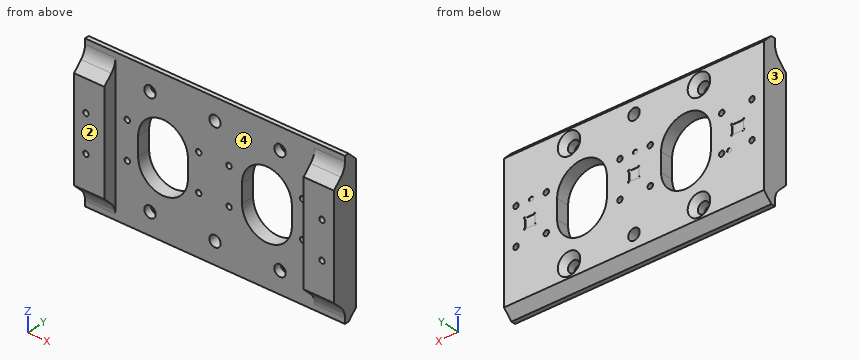
```python
from build123d import *

# Parameters (mm, degrees)
SKETCH_5_W                  = 120
SKETCH_5_H                  = 70
EXTRUDE_2_DEPTH             = 6
SKETCH1_R                   = 1
CUT_EXTRUDE1_DEPTH          = 0.2
SKETCH2_R                   = 1
CUT_EXTRUDE2_DEPTH          = 0.2
HOLE_WIZARD_M51_D           = 5.3
HOLE_WIZARD_M51_CSINK_D     = 10.4
HOLE_WIZARD_M51_CSINK_ANGLE = 90
SKETCH5_R                   = 2.6
CUT_EXTRUDE4_DEPTH          = 10
CUT_EXTRUDE4_TAPER          = -0.573055556
CUT_EXTRUDE_1_DEPTH         = 7.0000001
EXTRUDE_3_DEPTH             = 120
SKETCH_8_W                  = 92
SKETCH_8_H                  = 35.619722669
CUT_EXTRUDE_2_DEPTH         = 71
CHAMFER_1_SIZE              = 4
M3X0_51_D                   = 2.5


with BuildPart() as part:
    # Эскиз5 → Бобышка-Вытянуть2 (new body)
    with BuildSketch(Plane(origin=(0, 0, 0), x_dir=(1, 0, 0), z_dir=(0, 1, 0))):
        with Locations((60, 0)):
            Rectangle(SKETCH_5_W, SKETCH_5_H)
    extrude(amount=-EXTRUDE_2_DEPTH)

    # Sketch1 → Cut-Extrude1 (cut)
    with BuildSketch(Plane(origin=(0, 0, 0), x_dir=(1, 0, 0), z_dir=(0, 1, 0))):
        with Locations((16, 8)):
            Circle(SKETCH1_R)
        with BuildLine():
            Line((9.86, -2.16), (14.14, -2.16))
            ThreePointArc((14.14, -2.16), (14.993553391, -2.513553391), (14.64, -1.66))
            Line((14.64, -1.66), (14.64, 1.66))
            ThreePointArc((14.64, 1.66), (14.993553391, 2.513553391), (14.14, 2.16))
            Line((14.14, 2.16), (9.86, 2.16))
            ThreePointArc((9.86, 2.16), (9.006446609, 2.513553391), (9.36, 1.66))
            Line((9.36, 1.66), (9.36, -1.66))
            ThreePointArc((9.36, -1.66), (9.006446609, -2.513553391), (9.86, -2.16))
        make_face()
    extrude(amount=-CUT_EXTRUDE1_DEPTH, mode=Mode.SUBTRACT)

    # Sketch2 → Cut-Extrude2 (cut)
    with BuildSketch(Plane(origin=(0, 0, 0), x_dir=(1, 0, 0), z_dir=(0, 1, 0))):
        with Locations((59.481, -9.027)):
            Circle(SKETCH2_R)
        with Locations((107.481, -9.027)):
            Circle(SKETCH2_R)
        with BuildLine():
            Line((57.74, 1.76), (57.74, -1.76))
            ThreePointArc((57.74, -1.76), (57.386446609, -2.613553391), (58.24, -2.26))
            Line((58.24, -2.26), (61.76, -2.26))
            ThreePointArc((61.76, -2.26), (62.613553391, -2.613553391), (62.26, -1.76))
            Line((62.26, -1.76), (62.26, 1.76))
            ThreePointArc((62.26, 1.76), (62.613553391, 2.613553391), (61.76, 2.26))
            Line((61.76, 2.26), (58.24, 2.26))
            ThreePointArc((58.24, 2.26), (57.386446609, 2.613553391), (57.74, 1.76))
        make_face()
        with BuildLine():
            Line((105.74, 1.76), (105.74, -1.76))
            ThreePointArc((105.74, -1.76), (105.386446609, -2.613553391), (106.24, -2.26))
            Line((106.24, -2.26), (109.76, -2.26))
            ThreePointArc((109.76, -2.26), (110.613553391, -2.613553391), (110.26, -1.76))
            Line((110.26, -1.76), (110.26, 1.76))
            ThreePointArc((110.26, 1.76), (110.613553391, 2.613553391), (109.76, 2.26))
            Line((109.76, 2.26), (106.24, 2.26))
            ThreePointArc((106.24, 2.26), (105.386446609, 2.613553391), (105.74, 1.76))
        make_face()
    extrude(amount=-CUT_EXTRUDE2_DEPTH, mode=Mode.SUBTRACT)

    # Зенковка для  винта с плоской головкой M51 (through all)
    with Locations(Plane(origin=(0, 0, 0), x_dir=(1, 0, 0), z_dir=(0, 1, 0))):
        with Locations((30, 25), (90, 25), (90, -25), (30, -25)):
            CounterSinkHole(HOLE_WIZARD_M51_D / 2, HOLE_WIZARD_M51_CSINK_D / 2, counter_sink_angle=HOLE_WIZARD_M51_CSINK_ANGLE)

    # Sketch5 → Cut-Extrude4 (cut)
    with BuildSketch(Plane.XZ.offset(6)):
        with Locations((60, 25)):
            Circle(SKETCH5_R)
        with Locations((60, -25)):
            Circle(SKETCH5_R)
    extrude(amount=-CUT_EXTRUDE4_DEPTH, taper=CUT_EXTRUDE4_TAPER, mode=Mode.SUBTRACT)

    # Эскиз6 → Вырез-Вытянуть1 (cut, through all)
    with BuildSketch(Plane(origin=(0, 0, 0), x_dir=(1, 0, 0), z_dir=(0, 1, 0))):
        with BuildLine():
            Line((95.5, 4.35), (95.5, -4.35))
            ThreePointArc((95.5, -4.35), (84, -15.85), (72.5, -4.35))
            Line((72.5, -4.35), (72.5, 4.35))
            ThreePointArc((72.5, 4.35), (84, 15.85), (95.5, 4.35))
        make_face()
        with BuildLine():
            Line((47.5, 4.35), (47.5, -4.35))
            ThreePointArc((47.5, -4.35), (36, -15.85), (24.5, -4.35))
            Line((24.5, -4.35), (24.5, 4.35))
            ThreePointArc((24.5, 4.35), (36, 15.85), (47.5, 4.35))
        make_face()
    extrude(amount=-CUT_EXTRUDE_1_DEPTH, mode=Mode.SUBTRACT)

    # Эскиз7 → Бобышка-Вытянуть3 (add, through all)
    with BuildSketch(Plane.ZY):
        with BuildLine():
            Line((-32.5, -6), (32.5, -6))
            ThreePointArc((32.5, -6), (29.629874257, -6.570903506), (27.196699141, -8.196699141))
            Line((27.196699141, -8.196699141), (23.393398282, -12))
            Line((23.393398282, -12), (-23.393398282, -12))
            Line((-23.393398282, -12), (-27.196699141, -8.196699141))
            ThreePointArc((-27.196699141, -8.196699141), (-29.629874257, -6.570903506), (-32.5, -6))
        make_face()
    extrude(amount=-EXTRUDE_3_DEPTH)

    # Эскиз8 → Вырез-Вытянуть2 (cut, through all)
    with BuildSketch(Plane(origin=(0, 0, -35), x_dir=(-1, 0, 0), z_dir=(0, 0, -1))):
        with Locations((-60, -23.809861335)):
            Rectangle(SKETCH_8_W, SKETCH_8_H)
    extrude(amount=-CUT_EXTRUDE_2_DEPTH, mode=Mode.SUBTRACT)

    # Фаска1
    chamfer_1_edges = [part.edges().sort_by_distance(p)[0] for p in [
        (60, 0, 35),
        (60, 0, -35),
    ]]
    chamfer(chamfer_1_edges, length=CHAMFER_1_SIZE)

    # Отверстие обработанное метчиком M3x0.51 (through all)
    with Locations(Plane(origin=(0, 0, 0), x_dir=(1, 0, 0), z_dir=(0, 1, 0))):
        with Locations((114.481, -9.027), (100.481, -9.027), (100.481, 7.973), (114.481, 7.973), (66.481, 7.973), (52.481, 7.973), (52.481, -9.027), (66.481, -9.027), (19.5, -9), (5.5, -9), (5.5, 8), (19.5, 8)):
            Hole(M3X0_51_D / 2)


solid = part.part
```
Can you work these out from the model? Positions are in its coordinate system, mm. Face numbers are marked on the shaded views. Coordinates: 2 decimals unless noted, no trailing zeros. Loops run counter-clockwise (first coordinate to the right, second up) from the corner with the lowest first, then second, coordinate; pieces in that order, holes last. Notation, with made-up numbers: (21.5, 82.5) - (56.5, 82.5) arc R23 cw to (56.5, 101.5) - close; hole circle Ø2 at (61.25, 70.5). An arc over 180 degrees is marked (long way). Use a Markdown table: item, result.
Item 1: Will these pins go through, and if not, where does the flat tip stop? pin 1 (0.8 mm diameter, centred on x = 14.64, z = 2.16, fed in from -Y); pin 2 (8.5 mm diameter, centred on x = 90, z = 25, fed in from +Y).
Numbers:
| item | result |
|---|---|
| pin 1 | stops at y = -6 |
| pin 2 | stops at y = -0.95 |
Item 2: I want a section at D-D on x = 31.5. Give the number of separate pieces and of enclosed holes in the cut face, and give its area (3 significant figures).
Numbers:
| item | result |
|---|---|
| separate pieces | 4 |
| enclosed holes | 0 |
| area | 158 mm2 |
Item 3: I want a section at C-C on x = 71. Please give me the cut outline in (y, z).
Numbers:
| item | result |
|---|---|
| outline | (-6, -35) - (-4, -35) - (0, -31) - (0, 31) - (-4, 35) - (-6, 35) - close |
Item 4: If I drill on probe 1 along X at (y, z) = (-4.75, -3); probe 2 along Z at (x, y) = (5.5, -3.5); probe 3 along Z at (x, y) = (91, -2.5), over which ranges is the centre line in solid material (lowest first)? Write a range as from..to.
Numbers:
| item | result |
|---|---|
| probe 1 | x = 0..24.5, 47.5..72.5, 95.5..120 |
| probe 2 | z = -34.5..-9.25, -6.75..7.75, 10.25..34.5 |
| probe 3 | z = -33.5..-27.51, -22.49..-13.47, 13.47..22.49, 27.51..33.5 |
Item 5: We'd pull the mould along X, two halves only. Please class the marked faces 1, 2, 3 and 4: released by +X, released by -X, zero draft, split by the parting line, or undercut.
Numbers:
| item | result |
|---|---|
| face 1 | released by +X |
| face 2 | zero draft |
| face 3 | released by -X |
| face 4 | undercut |
Item 6: I want a section at A-A on x = 5.5. Please give me the cut outline in (y, z).
Numbers:
| item | result |
|---|---|
| outline | (-12, -23.39) - (-8.2, -27.2) arc R7.5 cw to (-6, -32.5) - (-6, -35) - (-4, -35) - (0, -31) - (0, -9.25) - (-12, -9.25) - close; (-12, -6.75) - (0, -6.75) - (0, 7.75) - (-12, 7.75) - close; (-12, 10.25) - (0, 10.25) - (0, 31) - (-4, 35) - (-6, 35) - (-6, 32.5) arc R7.5 cw to (-8.2, 27.2) - (-12, 23.39) - close |
Item 7: I want a section at B-B on x = 90. Please give me the cut outline in (y, z), and give its area (3 significant figures).
Numbers:
| item | result |
|---|---|
| outline | (-6, -35) - (-4, -35) - (0, -31) - (0, -30.2) - (-2.55, -27.65) - (-6, -27.65) - close; (-6, -22.35) - (-2.55, -22.35) - (0, -19.8) - (0, -14.16) - (-6, -14.16) - close; (-6, 14.16) - (0, 14.16) - (0, 19.8) - (-2.55, 22.35) - (-6, 22.35) - close; (-6, 27.65) - (-2.55, 27.65) - (0, 30.2) - (0, 31) - (-4, 35) - (-6, 35) - close |
| area | 157 mm2 |
